from build123d import *

# Parameters (mm, degrees)
SKETCH_1_R             = 5
EXTRUDE_1_DEPTH        = 56
SKETCH_2_R             = 6.5
EXTRUDE_2_DEPTH        = 4
HOLE_WIZARD_M6_1_D     = 5
HOLE_WIZARD_M6_1_DEPTH = 15
HOLE_WIZARD_M6_1_TIP   = 1.502151548


with BuildPart() as part:
    # 草图1 → 凸台-拉伸1 (new body)
    with BuildSketch(Plane.XY):
        Circle(SKETCH_1_R)
    extrude(amount=EXTRUDE_1_DEPTH)

    # 草图2 → 凸台-拉伸2 (add)
    with BuildSketch(Plane.XY.offset(56)):
        Circle(SKETCH_2_R)
    extrude(amount=EXTRUDE_2_DEPTH)

    # M6 螺纹孔1
    with Locations(Plane(origin=(0, 0, 0), x_dir=(-1, 0, 0), z_dir=(0, 0, -1))):
        with Locations((0, 0)):
            Hole(HOLE_WIZARD_M6_1_D / 2, depth=HOLE_WIZARD_M6_1_DEPTH)
            with Locations((0, 0, -(HOLE_WIZARD_M6_1_DEPTH + HOLE_WIZARD_M6_1_TIP / 2))):  # 118° drill point
                Cone(0, HOLE_WIZARD_M6_1_D / 2, HOLE_WIZARD_M6_1_TIP, mode=Mode.SUBTRACT)


solid = part.part
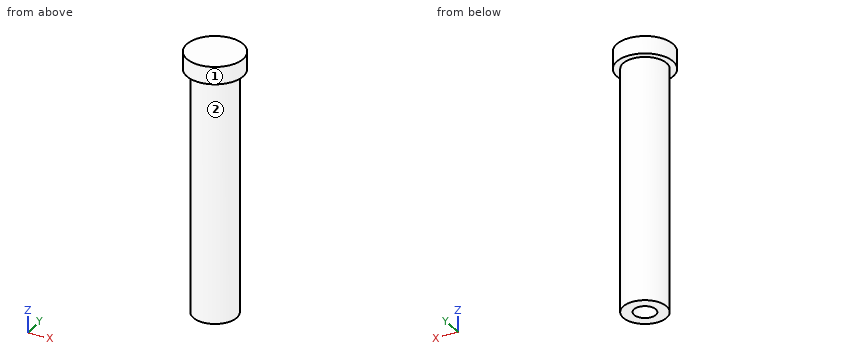
Model file for the job. Use its own axes, mm. Face numbers are marked on the shaded views. A direction names the side the tool comes from. Coordinates: 2 decimals unless noted, no trailing zeros. Write each loop counter-clockwise with the first axis right and the second up, starting at its lowest first coordinate (ties: lowest second). Pieces come first, ordered by that corner, then holes. Notation, with made-up numbers: (45.5, 59) -> (59.5, 59) arc R24 cw to (59.5, 85) -> close; hole circle Ø11 at (76, -10.5). An arc over 180 degrees is marked (long way). One line per item, written item: value. Start each with the question number.
1) Flat gauge pins, fed straight in: pin 1 Ø3 at (x, z) = (4, 8) entering from -Y; pin 2 Ø1.5 at (x, z) = (4.5, 43) entering from +Y; pin 3 Ø6.5 at (x, y) = (2.5, 0) entering from -Z; pin 4 Ø1 at (x, z) = (-2.5, 26) entering from -Y. Where does each tip first touch, or does it go through?
2) Slice it at D-D on x = -3.5. Write the cut outline in (y, z), then the cut area to 3 significant figures.
3) Slice it at B-B on x = 4. Write the cut outline in (y, z), then the cut area to 3 significant figures.
4) Probe probe 1 along Y at (x, z) = (0, 5.5); probe 2 along Y at (x, z) = (-1.5, 2.5); probe 3 along Z at (x, y) = (2.25, 6). List the from-to ranges inside material, lowest first.
5) Slice it at C-C on z = 21. Write the cut outline in (x, y), then the cut area to 3 significant figures.
6) Slice it at A-A on z = 12. Write the cut outline in (x, y), then the cut area to 3 significant figures.
7) Which spindle directions (+Z, -Z, +X, -X, +Y, -Y) get a long thin tool onto all of the face, cutting with end or side? Do the marked faces 1 and 2. Say none if no direction does.
Answers follow:
1. pin 1: y = -4.33
1. pin 2: y = 3.31
1. pin 3: z = 0
1. pin 4: y = -4.58
2. outline: (-5.48, 56) -> (-3.57, 56) -> (-3.57, 0) -> (3.57, 0) -> (3.57, 56) -> (5.48, 56) -> (5.48, 60) -> (-5.48, 60) -> close
2. area: 444 mm2
3. outline: (-5.12, 56) -> (-3, 56) -> (-3, 0) -> (3, 0) -> (3, 56) -> (5.12, 56) -> (5.12, 60) -> (-5.12, 60) -> close
3. area: 377 mm2
4. probe 1: -5 to -2.5, 2.5 to 5
4. probe 2: -4.77 to -2, 2 to 4.77
4. probe 3: 56 to 60
5. outline: circle Ø10 at (0, 0)
5. area: 78.5 mm2
6. outline: circle Ø10 at (0, 0); hole circle Ø5 at (0, 0)
6. area: 58.9 mm2
7. face 1: +Z, -Z
7. face 2: -Z
